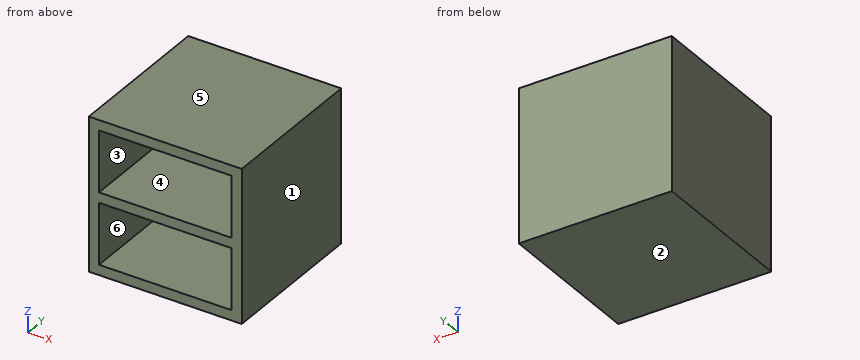
```python
from build123d import *

# Parameters (mm, degrees)
F0_W     = 180
F0_H     = 180
F1_DEPTH = 90
F2_T     = -12
F3_W     = 156
F3_H     = 12
F4_DEPTH = 168


with BuildPart() as f1:
    # F0 (on Top) → F1 (new body, symmetric)
    with BuildSketch(Plane.XY):
        Rectangle(F0_W, F0_H)
    extrude(amount=F1_DEPTH, both=True)

    # F2
    f2_openings = [f1.faces().sort_by_distance(p)[0] for p in [
        (0, -90, 0),
    ]]
    offset(amount=F2_T, openings=f2_openings)

    # F3 (on face) → F4 (join)
    with BuildSketch(Plane.XZ.offset(-78)):
        Rectangle(F3_W, F3_H)
    extrude(amount=F4_DEPTH)


solid = f1.part
```
Part model, mm, in its own coordinate system. Face numbers are marked on the shaded views. A direction names the side the tool comes from. Round coordinates to 2 decimals unless told otherwise and drop trailing zeros. Loops run counter-clockwise (first coordinate to the right, second up) from the corner with the lowest first, then second, coordinate; pieces in that order, holes last. Notation, with made-up numbers: (16, -37) -> (64, -37) arc R20 cw to (64, -19) -> close; hole circle Ø5 at (44, -28). An arc over 180 degrees is marked (long way). Use a Markdown table: item, result.
1) Tool access for the marked faces 5 and 6: list every direction of +Z, -Z, +X, -X, +Y, -Y with a clear straight run to the whole face (end or side of a thin tool).
The answers:
| item | result |
|---|---|
| face 5 | +Z, +X, -X, +Y, -Y |
| face 6 | -Y |
2) Pull direction X, two halves, no side cores. Call the marked faces 1, 2, 3 and 4: pulls with the +X half, pulls with the -X half, needs draft (parallel to the pull), parting line crosses it, or undercut.
The answers:
| item | result |
|---|---|
| face 1 | pulls with the +X half |
| face 2 | needs draft |
| face 3 | undercut |
| face 4 | undercut |
3) Cut at A-A, the plane y = -24.5. List the corners of the cut face in (x, z), and give its area (3 significant figures).
The answers:
| item | result |
|---|---|
| outline | (-90, -90) -> (90, -90) -> (90, 90) -> (-90, 90) -> close; hole (-78, -78) -> (78, -78) -> (78, -6) -> (-78, -6) -> close; hole (-78, 6) -> (78, 6) -> (78, 78) -> (-78, 78) -> close |
| area | 9,940 mm2 |
4) Drop a flat-ended pin along its axis: pin 1 Ø21.5 at (x, z) = (13.5, -33) entering from -Y. Give the stop position or say it passes through.
The answers:
| item | result |
|---|---|
| pin 1 | stops at y = 78 |
5) Cut at B-B, the plane z = -29.5. List the corners of the cut face in (x, y).
The answers:
| item | result |
|---|---|
| outline | (-90, -90) -> (-78, -90) -> (-78, 78) -> (78, 78) -> (78, -90) -> (90, -90) -> (90, 90) -> (-90, 90) -> close |
6) Cut at C-C, the plane x = -4. List the corners of the cut face in (y, z), and give its area (3 significant figures).
The answers:
| item | result |
|---|---|
| outline | (-90, -90) -> (90, -90) -> (90, 90) -> (-90, 90) -> (-90, 78) -> (78, 78) -> (78, 6) -> (-90, 6) -> (-90, -6) -> (78, -6) -> (78, -78) -> (-90, -78) -> close |
| area | 8,210 mm2 |
7) Probe line 1 (Z direction, x = 53.5, y = -4); line 2 (X direction, y = -62.5, z = 47); line 3 (Y direction, x = -42.5, z = -29). List the from-to ranges inside material, lowest first. Write a range as [from, to].
The answers:
| item | result |
|---|---|
| line 1 | z = [-90, -78], [-6, 6], [78, 90] |
| line 2 | x = [-90, -78], [78, 90] |
| line 3 | y = [78, 90] |
